```python
from build123d import *

# Parameters (mm, degrees)
F0_R     = 25
F0_R_2   = 19.066290696
F1_DEPTH = 25
F0_R_3   = 40
F0_R_4   = 2.5
F2_DEPTH = 10
F3_R     = 4.99999
F4_R     = 4.99999


# Not quite as in the source:
# - a fillet or chamfer is up to 0.001 mm smaller than in the source, because OpenCascade refuses the exact size


with BuildPart() as f1:
    # F0 (on Top) → F1 (new body)
    with BuildSketch(Plane.XY):
        Circle(F0_R)
        Circle(F0_R_2, mode=Mode.SUBTRACT)
    extrude(amount=F1_DEPTH)

    # F0 (on Top) → F2 (join)
    with BuildSketch(Plane.XY):
        Circle(F0_R_3)
        with Locations((-32.5, 0)):
            Circle(F0_R_4, mode=Mode.SUBTRACT)
        Circle(F0_R, mode=Mode.SUBTRACT)
        with Locations((32.5, 0)):
            Circle(F0_R_4, mode=Mode.SUBTRACT)
    extrude(amount=F2_DEPTH)

    # F3 (radius 5 in the source; OpenCascade refuses exactly that, so slightly less here)
    f3_edges = [f1.edges().sort_by_distance(p)[0] for p in [
        (-40, 0, 10),
        (-25, 0, 25),
    ]]
    fillet(f3_edges, radius=F3_R)

    # F4 (radius 5 in the source; OpenCascade refuses exactly that, so slightly less here)
    f4_edges = [f1.edges().sort_by_distance(p)[0] for p in [
        (25, 0, 15.000005),
        (-25, 0, 20.00001),
        (-25, 0, 10),
    ]]
    fillet(f4_edges, radius=F4_R)


solid = f1.part
```
The model under review builds one solid part; all positions refer to its coordinate system, in mm. Round coordinates to 2 decimals unless told otherwise and drop trailing zeros. Write each loop counter-clockwise with the first axis right and the second up, starting at its lowest first coordinate (ties: lowest second). Pieces come first, ordered by that corner, then holes.
(1) Wall thickness on L1, parallel to Y at x = 0, z = 16.5; L2, parallel to Z at x = 30, y = -1; L3, parallel to Y at x = -32.5, z = 6.25: over which ranges is each line inside the solid? List them lowest first.
(2) We need section A-A on y = 0. Give the number of separate pieces and of enclosed holes in the cut face, and give its area (3 significant figures).
(3) We need section B-B on x = 0. Give the boundary of the cut face in (y, z), and give its area (3 significant figures).
(4) Mouldability with a two-part tool opening along Y and no side actions: class faces 1 (the cylindrical face through (-35, 0, 5)), 2 (the flat face through (10.2, -28.4, 10)), 3 (the cylindrical face through (23.846, 7.509, 17.465)) as +Y half, -Y half, draft (parallel to the pull), parting line (faces both ways), or undercut.
(5) Insertion check: pin 1 (1.5 mm diameter, centred on x = 8, z = 6.5, fed in from -Y); pin 2 (8 mm diameter, centred on y = 10.5, z = 13.5, fed in from +X); pin 3 (6 mm diameter, centred on x = -20.5, z = 5, fed in from -Y). Each pin has a flat end and moves straight along its axis. Give the tip position at first contact, or say it passes through.
Findings below:
1. L1: y = -25 to -19.07, 19.07 to 25
1. L2: z = 0 to 10
1. L3: y = -23.05 to -2.5, 2.5 to 23.05
2. separate pieces: 4
2. enclosed holes: 0
2. area: 486 mm2
3. outline: (-40, 0) - (-19.07, 0) - (-19.07, 25) - (-20, 25) arc R5 ccw to (-25, 20) - (-25, 15) arc R5 cw to (-30, 10) - (-35, 10) arc R5 ccw to (-40, 5) - close; (19.07, 0) - (40, 0) - (40, 5) arc R5 ccw to (35, 10) - (30, 10) arc R5 cw to (25, 15) - (25, 20) arc R5 ccw to (20, 25) - (19.07, 25) - close
3. area: 586 mm2
4. face 1: undercut
4. face 2: draft
4. face 3: parting line
5. pin 1: stops at y = -39.2
5. pin 2: stops at x = 35.74
5. pin 3: stops at y = -35.97
